Check sheet for the drawn part. Datum: minimum x, y, z corner. Units: mm. A direction names the side the tool comes from. Round coordinates to 2 decimals unless told otherwise and drop trailing zeros. Loops run counter-clockwise (first coordinate to the right, second up) from the corner with the lowest first, then second, coordinate; pieces in that order, holes last.
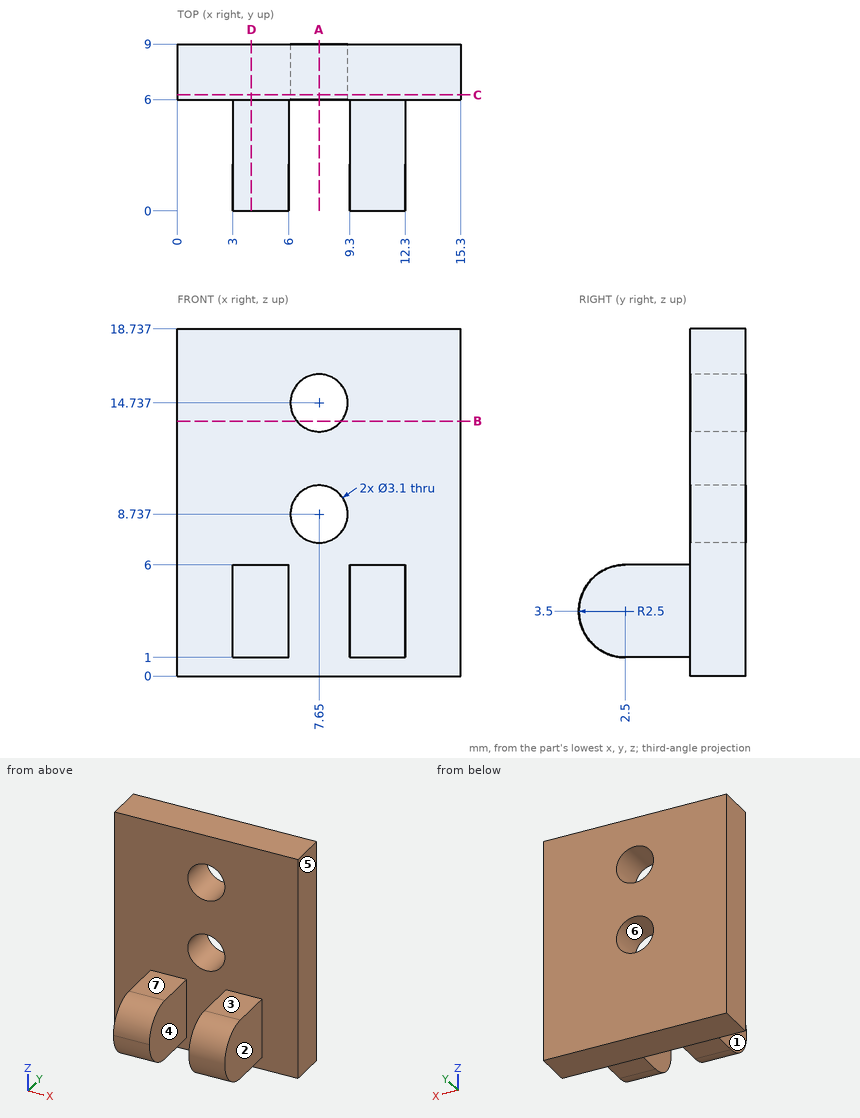
1) Sectioned sample at A-A, the plane x = 7.65. Record the cut outline in (y, z).
Report:
outline: (6, 0) - (9, 0) - (9, 7.19) - (6, 7.19) - close; (6, 10.29) - (9, 10.29) - (9, 13.19) - (6, 13.19) - close; (6, 16.29) - (9, 16.29) - (9, 18.74) - (6, 18.74) - close
2) Scan lines: line 1 along Z through (x, y) = (7.65, 8.4); line 2 along X through (y, z) = (2, 2.5); line 3 along Y through (x, z) = (13.5, 13.5). Record each from-to range of solid material in increasing order.
Report:
line 1: z = 0 to 7.19, 10.29 to 13.19, 16.29 to 18.74
line 2: x = 3 to 6, 9.3 to 12.3
line 3: y = 6 to 9
3) Sectioned sample at B-B, the plane z = 13.75. Record the cut outline in (x, y) (1 decimal).
Report:
outline: (0, 6) - (6.5, 6) - (6.5, 9) - (0, 9) - close; (8.8, 6) - (15.3, 6) - (15.3, 9) - (8.8, 9) - close
4) Mould release check, pull along X, two halves, no side actions. Record for the marked faces 5, 6 and 7: +X half, -X half, draft (parallel to the pull), parting line (faces both ways), or undercut.
Report:
face 5: +X half
face 6: undercut
face 7: draft
5) Sectioned sample at C-C, the plane y = 6.25. Record the cut outline in (x, z).
Report:
outline: (0, 0) - (15.3, 0) - (15.3, 18.74) - (0, 18.74) - close; hole circle Ø3.1 at (7.65, 8.74); hole circle Ø3.1 at (7.65, 14.74)
6) Sectioned sample at D-D, the plane x = 4. Record the cut outline in (y, z).
Report:
outline: (2.5, 1) - (6, 1) - (6, 0) - (9, 0) - (9, 18.74) - (6, 18.74) - (6, 6) - (2.5, 6) arc R2.5 ccw to start
7) Access from +Z, -Z, +X, -X, +Y, -Y to the whole of each face (thin tool, end or side, straight path). Record for the marked faces 1, 2, 3 and 4.
Report:
face 1: +Z, -Z, -X, -Y
face 2: +Z, -Z, +X, -Y
face 3: +Z, +X, -X, -Y
face 4: +Z, -Z, -Y
8) Gauge pin test, flat ends, axial feed: pin 1 (0.9 mm diameter, centred on x = 4.5, y = 3.5, fed in from +Z); pin 2 (2.5 mm diameter, centred on y = 4, z = 3, fed in from -X); pin 3 (3 mm diameter, centred on x = 7.65, z = 8.74, fed in from +Y); pin 4 (0.9 mm diameter, centred on x = 4, y = 4, fed in from -Z). Record the tip position at first contact, or that the pin passes through.
Report:
pin 1: stops at z = 6
pin 2: stops at x = 3
pin 3: passes through
pin 4: stops at z = 1
